Source: CAD feature listing. Evaluate the final solid. Frame: model axes, mm. A direction names the side the tool comes from. Coordinates: 2 decimals unless noted, no trailing zeros. Write each loop counter-clockwise with the first axis right and the second up, starting at its lowest first coordinate (ties: lowest second). Pieces come first, ordered by that corner, then holes. Notation, with made-up numbers: M -14.75,-26 L 13.25,-26 A23 cw 13.25,-1 Z; hole C 9.5,77 d3. An arc over 180 degrees is marked long. One line per item, written item: value. Start each with the question number.
Item 1: Set-up query: faces 1 (the flat face through (-3, 56, -27)), 2 (the cylindrical face through (-882.712, 43.51, -54.26)), 3 (the flat face through (-710, 54, -55)). Return all of +Z, -Z, +X, -X, +Y, -Y with unobstructed straight access to the full face (end or side cutting, diameter ignored); none if empty.
Item 2: Mould query, pull axis Y, two halves, no side actions, for faces 4 (the flat face through (0, 54, -27)), 5 (the flat face through (-710, 110, -28)), 6 (the cylindrical face through (-46.793, 65.814, -0.74)). Classes: released by +Y, released by -Y, zero draft, split by the parting line, or undercut.
Item 3: Cut plane B-B, the plane z = -24.5. Output: boundary loops of the cut face in (x, y), then the cut area to 3 significant figures.
Item 4: Pin query (flat end, axial travel): P1, Ø1.5, axis at x = -924.5, y = 66, coming from the +Z side; P2, Ø5, axis at x = -230.5, y = 81.5, coming from the -Z side. Return the tip coordinate at first contact, or that it passes through.
Item 5: Cut plane C-C, the plane x = -330. Output: boundary loops of the cut face in (y, z).
Item 6: Ray query, L1, parallel to X at y = 81, z = -8; L2, parallel to Y at x = -1100.5, z = -4; L3, parallel to Z at x = -852, y = 87.5. Return the intervals inside material, ascending. Write a range as from..to.
Item 7: Cut plane A-A, the plane x = -476.5. Output: boundary loops of the cut face in (y, z), then the cut area to 3 significant figures.
```python
from build123d import *

# Parameters (mm, degrees)
SKETCH_1_W          = 1400
SKETCH_1_H          = 55
EXTRUDE_1_DEPTH     = 110
SKETCH_3_R          = 30
SKETCH_3_R_2        = 2.5
CUT_EXTRUDE_1_DEPTH = 10
CUT_EXTRUDE_START   = -3
SKETCH_4_W          = 52
SKETCH_4_H          = 107
CUT_EXTRUDE_2_DEPTH = 1394
SKETCH_5_R          = 16
CUT_EXTRUDE_3_DEPTH = 10


with BuildPart() as part:
    # Эскиз1 → Бобышка-Вытянуть1 (new body)
    with BuildSketch(Plane(origin=(0, 0, 0), x_dir=(1, 0, 0), z_dir=(0, 1, 0))):
        with Locations((-700, 27.5)):
            Rectangle(SKETCH_1_W, SKETCH_1_H)
    extrude(amount=EXTRUDE_1_DEPTH)

    # Эскиз3 → Вырез-Вытянуть1 (cut)
    with BuildSketch(Plane(origin=(0, 0, -55), x_dir=(-1, 0, 0), z_dir=(0, 0, -1))):
        with Locations((120, 55)):
            Circle(SKETCH_3_R)
        with Locations((225, 55)):
            Circle(SKETCH_3_R)
        with Locations((330, 55)):
            Circle(SKETCH_3_R)
        with Locations((435, 55)):
            Circle(SKETCH_3_R)
        with Locations((540, 55)):
            Circle(SKETCH_3_R)
        with Locations((645, 55)):
            Circle(SKETCH_3_R)
        with Locations((750, 55)):
            Circle(SKETCH_3_R)
        with Locations((855, 55)):
            Circle(SKETCH_3_R)
        with Locations((960, 55)):
            Circle(SKETCH_3_R)
        with Locations((1380, 55)):
            Circle(SKETCH_3_R_2)
        with Locations((1065, 55)):
            Circle(SKETCH_3_R)
        with Locations((1170, 55)):
            Circle(SKETCH_3_R)
        with Locations((1275, 55)):
            Circle(SKETCH_3_R)
    extrude(amount=-CUT_EXTRUDE_1_DEPTH, mode=Mode.SUBTRACT)

    # Эскиз4 → Вырез-Вытянуть2 (cut)
    with BuildSketch(Plane(origin=(0, 0, 0), x_dir=(0, 0, -1), z_dir=(1, 0, 0)).offset(CUT_EXTRUDE_START)):
        with Locations((27.5, 55)):
            Rectangle(SKETCH_4_W, SKETCH_4_H)
    extrude(amount=-CUT_EXTRUDE_2_DEPTH, mode=Mode.SUBTRACT)

    # Эскиз5 → Вырез-Вытянуть3 (cut)
    with BuildSketch(Plane.XY):
        with Locations((-35, 55)):
            Circle(SKETCH_5_R)
    extrude(amount=-CUT_EXTRUDE_3_DEPTH, mode=Mode.SUBTRACT)


solid = part.part
```
From the geometry:
1. face 1: none
1. face 2: -Z
1. face 3: -Z, +X, -X, +Y, -Y
2. face 4: zero draft
2. face 5: released by +Y
2. face 6: undercut
3. outline: M -1400,0 L 0,0 L 0,110 L -1400,110 Z; hole M -1397,1.5 L -3,1.5 L -3,108.5 L -1397,108.5 Z
3. area: 4,840 mm²
4. P1: stops at z = 0
4. P2: stops at z = -1.5
5. outline: M 0,-55 L 25,-55 L 25,-53.5 L 1.5,-53.5 L 1.5,-1.5 L 108.5,-1.5 L 108.5,-53.5 L 85,-53.5 L 85,-55 L 110,-55 L 110,0 L 0,0 Z
6. L1: x = -1400..-1397, -3..0
6. L2: y = 0..1.5, 108.5..110
6. L3: z = -55..-53.5, -1.5..0
7. outline: M 0,-55 L 110,-55 L 110,0 L 0,0 Z; hole M 1.5,-53.5 L 108.5,-53.5 L 108.5,-1.5 L 1.5,-1.5 Z
7. area: 486 mm²
